```python
from build123d import *

# Parameters (mm, degrees)
SKETCH1_R           = 2.5
SKETCH1_R_2         = 3.57
BOSS_EXTRUDE1_DEPTH = 6


with BuildPart() as part:
    # Sketch1 → Boss-Extrude1 (new, symmetric)
    with BuildSketch(Plane.XY):
        with BuildLine():
            Line((-39.64, -10), (39.64, -10))
            ThreePointArc((39.64, -10), (42.015878785, -9.015878785), (43, -6.64))
            Line((43, -6.64), (43, 6.64))
            ThreePointArc((43, 6.64), (42.015878785, 9.015878785), (39.64, 10))
            Line((39.64, 10), (-39.64, 10))
            ThreePointArc((-39.64, 10), (-42.015878785, 9.015878785), (-43, 6.64))
            Line((-43, 6.64), (-43, -6.64))
            ThreePointArc((-43, -6.64), (-42.015878785, -9.015878785), (-39.64, -10))
        make_face()
        with Locations((-30, 0)):
            Circle(SKETCH1_R, mode=Mode.SUBTRACT)
        Circle(SKETCH1_R_2, mode=Mode.SUBTRACT)
        with Locations((30, 0)):
            Circle(SKETCH1_R, mode=Mode.SUBTRACT)
        with Locations((-20, 0)):
            Circle(SKETCH1_R, mode=Mode.SUBTRACT)
        with Locations((20, 0)):
            Circle(SKETCH1_R, mode=Mode.SUBTRACT)
    extrude(amount=BOSS_EXTRUDE1_DEPTH, both=True)


solid = part.part
```
CAD build for the part. Positions are in the model's coordinates, mm. Round coordinates to 2 decimals unless told otherwise and drop trailing zeros. Loops run counter-clockwise (first coordinate to the right, second up) from the corner with the lowest first, then second, coordinate; pieces in that order, holes last. Notation, with made-up numbers: M 85,33.25 L 125,33.25 A26 ccw 125,61.25 Z; hole C -19.75,88.5 d10. An arc over 180 degrees is marked long. Return JSON: item names as keys, results as strings. Group by question number.
(1) Saw through at B-B, the plane x = -20. List the corners of the cut face in (y, z).
(2) Drop a flat-ended pin along its axis: P1, Ø1.5, axis at x = 30, y = 0.5, coming from the -Z side. Give the stop position or say it passes through.
(3) Wall check: probe 1 along Y at (x, z) = (20, -3); probe 2 along X at (y, z) = (2.25, -2.25); probe 3 along Y at (x, z) = (0, -3). Give the ranges that are in metal, low to high. Write a range as [from, to].
(4) Mould opens along X. For faces 1 (the flat face through (1, 10, 0)), 2 (the cylindrical face through (17.5, 0.1, -0.1)), 3 (the cylindrical face through (-32.5, 0.1, -0.1)), 4 (the flat face through (43, 0, 0)) say: +X half, -X half, draft (parallel to the pull), parting line (faces both ways), or undercut.
(5) Saw through at A-A, the plane y = 0. List the corners of the cut face in (x, z), and give its area (3 significant figures).
(6) Saw through at C-C, the plane z = 4.5. List the corners of the cut face in (x, y).
Answer list:
{
 "1": {"outline": "M -10,-6 L -2.5,-6 L -2.5,6 L -10,6 Z; M 2.5,-6 L 10,-6 L 10,6 L 2.5,6 Z"},
 "2": {"P1": "through"},
 "3": {"probe 1": "[-10, -2.5], [2.5, 10]", "probe 2": "[-43, -31.09], [-28.91, -21.09], [-18.91, -2.77], [2.77, 18.91], [21.09, 28.91], [31.09, 43]", "probe 3": "[-10, -3.57], [3.57, 10]"},
 "4": {"face 1": "draft", "face 2": "undercut", "face 3": "undercut", "face 4": "+X half"},
 "5": {"outline": "M -43,-6 L -32.5,-6 L -32.5,6 L -43,6 Z; M -27.5,-6 L -22.5,-6 L -22.5,6 L -27.5,6 Z; M -17.5,-6 L -3.57,-6 L -3.57,6 L -17.5,6 Z; M 3.57,-6 L 17.5,-6 L 17.5,6 L 3.57,6 Z; M 22.5,-6 L 27.5,-6 L 27.5,6 L 22.5,6 Z; M 32.5,-6 L 43,-6 L 43,6 L 32.5,6 Z", "area": "706 mm2"},
 "6": {"outline": "M -43,-6.64 A3.36 ccw -39.64,-10 L 39.64,-10 A3.36 ccw 43,-6.64 L 43,6.64 A3.36 ccw 39.64,10 L -39.64,10 A3.36 ccw -43,6.64 Z; hole C -30,0 d5; hole C -20,0 d5; hole C 0,0 d7.14; hole C 20,0 d5; hole C 30,0 d5"}
}
